Can you work these out from the model? Positions are in its coordinate system, mm. Face numbers are marked on the shaded views. A direction names the side the tool comes from. Give positions to 0.01 mm unless a question says otherwise; leave off trailing zeros. Answer as CSV lines item,"result". Start each with the question number.
1. On a 3-axis mill with a long thin cutter (end or side, diameter ignored), from which of +Z, -Z, +X, -X, +Y, -Y can I reach the whole of each face in a straight line? I mean the marked faces 1, 2 and 3. Say none if no direction works.
2. I need wall thicknesses on line 1 (Z direction, x = -20, y = -4.25); line 2 (Z direction, x = -23.5, y = -11); line 3 (X direction, y = -5, z = 16). Which ranges of each line are inside material? Lowest first, please. Write a range as [from, to].
3. I'm going to push flat-ended pins straight in: P1, Ø7.5, axis at x = -25, z = 15, coming from the -Y side; P2, Ø4, axis at y = -5.5, z = 28.5, coming from the -X side; P3, Ø12, axis at y = -11.5, z = 12, coming from the +X side. Where does each tip first touch, or does it pass through?
4. If we section it at A-A on z = 9.5: Count the separate pieces of the cut face and the enclosed holes in it, plus the area to 3 significant figures.
5. If we mould it in two halves opening along X, with no side actions, what happens to the marked faces 4, 5, 6 and 7? For each: pulls with the +X half, pulls with the -X half, needs draft (parallel to the pull), parting line crosses it, or undercut.
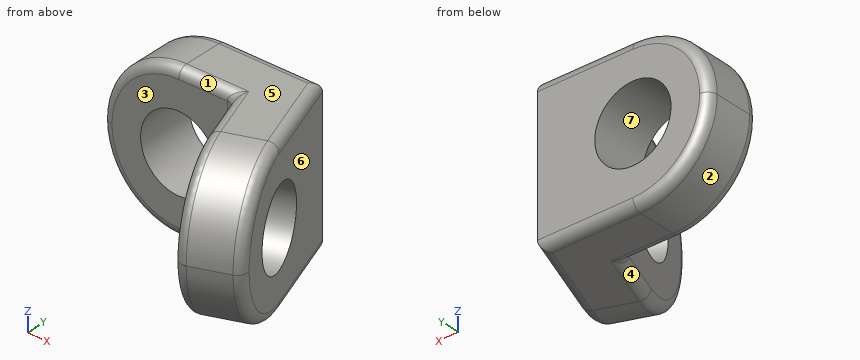
Autodesk Inventor part; units mm, degrees
ref_plane "YZ Plane" through (0, 0, 0) normal (1, 0, 0) x (0, 1, 0)
ref_plane "XZ Plane" through (0, 0, 0) normal (0, 1, 0) x (-1, 0, 0)
ref_plane "XY Plane" through (0, 0, 0) normal (0, 0, 1) x (1, 0, 0)
sketch "Sketch1" plane through (0, 0, 0) normal (0, 0, 1) x (1, 0, 0)
  line L0 (0, -45.5198) -> (0, 7.5866)
  line L1 (-45.6625, 0) -> (21.9753, 0)
  line L2 (0, 0) -> (-36, 0)
  line L3 (-36, 0) -> (-36, -12)
  line L4 (-36, -12) -> (-8.4025, -12)
  line L5 (-8.4025, -12) -> (0, 0) construction
  line L6 (0, 0) -> (12.3127, -33.8289)
  line L7 (12.3127, -33.8289) -> (1.0364, -37.9332)
  line L8 (1.0364, -37.9332) -> (-8.4025, -12)
  dimension "d0" = 36
  dimension "d1" = 12
  dimension "d2" = 55
extrude "Extrusion1" add sketch "Sketch1" along normal blind 32
fillet "Fillet1" radius 16 4 edges at (-36, -6, 32) (6.6746, -35.8811, 32) (6.6746, -35.8811, 0) (-36, -6, 0)
hole "Hole1" at (-20, -12, 16) direction (0, 1, 0) diameter 16 end through all
hole "Hole2" at (-4.4359, -22.8981, 16) direction (0.9396926, 0.3420201, 0) diameter 16 end through all
fillet "Fillet2" radius 2 12 edges at (3.4202, -9.397, 32) (10.7099, -29.4253, 27.3137) (3.4202, -9.397, 0) (-6.4192, -17.4491, 32) (-0.5664, -33.5295, 27.3137) (-6.4192, -17.4491, 0) (-14.2013, -12, 32) (-31.3137, -12, 27.3137) (-14.2013, -12, 0) (-10.0001, 0, 32) (-31.3137, 0, 27.3137) (-10.0001, 0, 0)
fillet "Fillet3" radius 2 3 edges at (-8.4025, -12, 16) (-7.9923, -11.4142, 31.4142) (-7.9923, -11.4142, 0.5858)
properties part number "Levier"
Computed values:
1,face 1,"+Z, -X, -Y"
1,face 2,"-Z, -X, +Y, -Y"
1,face 3,"+Z, -Z, -X, -Y"
2,line 1,"z = [0, 8], [24, 32]"
2,line 2,"z = [0.66, 8.81], [23.19, 31.34]"
2,line 3,"x = [-36, -28], [-12, 1.82]"
3,P1,"stops at y = -12"
3,P2,"stops at x = -32.07"
3,P3,"stops at x = 5.94"
4,separate pieces,"3"
4,enclosed holes,"0"
4,area,"503 mm2"
5,face 4,"pulls with the -X half"
5,face 5,"needs draft"
5,face 6,"pulls with the +X half"
5,face 7,"undercut"
